Can you work these out from the model? Positions are in its coordinate system, mm. A direction names the side the tool comes from. Give positions to 0.01 mm unless a question says otherwise; leave off trailing zeros. Write each loop counter-clockwise with the first axis right and the second up, starting at its lowest first coordinate (ties: lowest second). Pieces come first, ordered by that corner, then holes. Notation, with made-up numbers: (16.5, 87.5) - (48.5, 87.5) arc R27 cw to (48.5, 117.5) - close; hole circle Ø8 at (58, 63). An arc over 180 degrees is marked (long way). Use a Markdown table: item, result. Add a question column.
```python
from build123d import *

# Parameters (mm, degrees)
SKETCH3_R           = 3.175
BOSS_EXTRUDE1_DEPTH = 25.4
CIRPATTERN3_COUNT   = 5


with BuildPart() as part:
    # Sketch1 → Revolve1 (revolve)
    with BuildSketch(Plane.XY):
        Polygon((0, 25.4), (12.7, 25.4), (12.7, 50.8), (19.05, 50.8), (19.05, 25.4), (50.8, 25.4), (50.8, 22.225), (47.625, 22.225), (47.625, 12.7), (3.175, 12.7), (3.175, 22.225), (0, 22.225), align=None)
    revolve(axis=Axis((0, 0, 0), (1, 0, 0)))

    # Sketch3 → Boss-Extrude1 (add)
    with BuildSketch(Plane(origin=(19.05, 0, 0), x_dir=(0, 0, -1), z_dir=(1, 0, 0))):
        with Locations((0, 38.1)):
            Circle(SKETCH3_R)
    boss_extrude1 = extrude(amount=BOSS_EXTRUDE1_DEPTH)

    # CirPattern3: Boss-Extrude1 ×5 about axis
    cirpattern3_axis = Axis((0, 0, 0), (1, 0, 0))
    for i in range(1, CIRPATTERN3_COUNT):
        add(boss_extrude1.rotate(cirpattern3_axis, i * 360 / CIRPATTERN3_COUNT))


solid = part.part
```
Q1. On a 3-axis mill with a long thin cutter (end or side, diameter ignored), from which of +Z, -Z, +X, -X, +Y, -Y can I reach the whole of each face in a straight line? I mean faces 1 (the flat face through (44.45, 12, -36)), 2 (the flat face through (12.7, -10.6, 23.3)), 3 (the flat face through (44.45, 12, 36)). Say none if no direction works.
Q2. Suppose I cut it at D-D (z = 16). Please give me the cut outline in (x, y) (3 decimals), and give its area (3 significant figures).
Q3. Suppose I cut it at A-A (y = 0). Please give me the cut outline in (x, z) (3 decimals), and give its area (3 significant figures).
Q4. I'm going to push flat-ended pins straight in: P1, Ø4, axis at y = -21, z = 38, coming from the +X side; P2, Ø7, axis at y = 12, z = -37.5, coming from the +X side; P3, Ø13.5, axis at y = 7, z = -11, coming from the -X side (3 decimals). Where does each tip first touch, or does it pass through?
Q5. Suppose I cut it at B-B (z = 0). Please give me the cut outline in (x, y) (3 decimals), and give its area (3 significant figures).
Q6. Suppose I cut it at C-C (x = 27). Please give me the cut outline in (y, z) (3 decimals).
Q7. If we mould it in two halves opening along Y, with no side actions, what happens to faces 4 (the cylindrical face through (31.57, 10.98, -39.31)), 5 (the cylindrical face through (31.57, -27.78, -23.3)), 6 (the cylindrical face through (35.147, -5.506, -24.796)), 7 (the flat face through (44.45, -31, -22))? For each: released by +Y, released by -Y, zero draft, split by the parting line, or undercut.
Q8. If I drill on probe 1 along Z at (x, y) = (50, 0) (3 decimals); probe 2 along Z at (x, y) = (33, 0); probe 3 along X at (y, z) = (-30.5, -13), over which ranges is the centre line in solid material (lowest first)? Write a range as [from, to].
Derived:
| question | item | result |
|---|---|---|
| 1 | face 1 | -Z, +X, +Y, -Y |
| 1 | face 2 | -X |
| 1 | face 3 | +Z, +X, +Y, -Y |
| 2 | outline | (0, -19.727) - (12.7, -19.727) - (12.7, -48.215) - (19.05, -48.215) - (19.05, -19.727) - (50.8, -19.727) - (50.8, -15.426) - (47.625, -15.426) - (47.625, 15.426) - (50.8, 15.426) - (50.8, 19.727) - (19.05, 19.727) - (19.05, 48.215) - (12.7, 48.215) - (12.7, 19.727) - (0, 19.727) - (0, 15.426) - (3.175, 15.426) - (3.175, -15.426) - (0, -15.426) - close |
| 2 | area | 2,170 mm² |
| 3 | outline | (0, -25.4) - (12.7, -25.4) - (12.7, -50.8) - (19.05, -50.8) - (19.05, -25.4) - (50.8, -25.4) - (50.8, -22.225) - (47.625, -22.225) - (47.625, -12.7) - (3.175, -12.7) - (3.175, -22.225) - (0, -22.225) - close; (0, 22.225) - (3.175, 22.225) - (3.175, 12.7) - (47.625, 12.7) - (47.625, 22.225) - (50.8, 22.225) - (50.8, 25.4) - (19.05, 25.4) - (19.05, 50.8) - (12.7, 50.8) - (12.7, 25.4) - (0, 25.4) - close |
| 3 | area | 1,490 mm² |
| 4 | P1 | x = 19.05 |
| 4 | P2 | x = 44.45 |
| 4 | P3 | x = 3.175 |
| 5 | outline | (0, -25.4) - (12.7, -25.4) - (12.7, -50.8) - (19.05, -50.8) - (19.05, -25.4) - (50.8, -25.4) - (50.8, -22.225) - (47.625, -22.225) - (47.625, -12.7) - (3.175, -12.7) - (3.175, -22.225) - (0, -22.225) - close; (0, 22.225) - (3.175, 22.225) - (3.175, 12.7) - (47.625, 12.7) - (47.625, 22.225) - (50.8, 22.225) - (50.8, 25.4) - (19.05, 25.4) - (19.05, 34.925) - (44.45, 34.925) - (44.45, 41.275) - (19.05, 41.275) - (19.05, 50.8) - (12.7, 50.8) - (12.7, 25.4) - (0, 25.4) - close |
| 5 | area | 1,650 mm² |
| 6 | outline | circle Ø6.35 at (-30.824, -22.395); circle Ø6.35 at (-30.824, 22.395); circle Ø50.8 at (0, 0); circle Ø6.35 at (11.774, -36.235); circle Ø6.35 at (11.774, 36.235); circle Ø6.35 at (38.1, 0); hole circle Ø25.4 at (0, 0) |
| 7 | face 4 | split by the parting line |
| 7 | face 5 | undercut |
| 7 | face 6 | undercut |
| 7 | face 7 | zero draft |
| 8 | probe 1 | [-25.4, -22.225], [22.225, 25.4] |
| 8 | probe 2 | [-25.4, -12.7], [12.7, 25.4] |
| 8 | probe 3 | [12.7, 19.05] |
